Geometry check sheet. Reference: the model listing, model coordinates, mm. A direction names the side the tool comes from. Coordinates: 2 decimals unless noted, no trailing zeros. Write each loop counter-clockwise with the first axis right and the second up, starting at its lowest first coordinate (ties: lowest second). Pieces come first, ordered by that corner, then holes. Notation, with made-up numbers: (78, -26.75) -> (124, -26.75) arc R18 ccw to (124, -8.75) -> close; hole circle Ø3 at (26.5, 67.25). An arc over 180 degrees is marked (long way). Answer as CSV lines item,"result".
```python
from build123d import *

# Parameters (mm, degrees)
SKETCH1_W           = 42
SKETCH1_H           = 20
BOSS_EXTRUDE1_DEPTH = 42
SKETCH2_W           = 55
SKETCH2_H           = 3
BOSS_EXTRUDE2_DEPTH = 20
SKETCH3_R           = 1
CUT_EXTRUDE1_DEPTH  = 42
SKETCH4_R           = 3
BOSS_EXTRUDE3_DEPTH = 5


with BuildPart() as part:
    # Sketch1 → Boss-Extrude1 (new body)
    with BuildSketch(Plane(origin=(0, 0, 0), x_dir=(1, 0, 0), z_dir=(0, 1, 0))):
        with Locations((21, 10)):
            Rectangle(SKETCH1_W, SKETCH1_H)
    extrude(amount=BOSS_EXTRUDE1_DEPTH)

    # Sketch2 → Boss-Extrude2 (add)
    with BuildSketch(Plane.XY):
        with Locations((21, 31.5)):
            Rectangle(SKETCH2_W, SKETCH2_H)
    extrude(amount=-BOSS_EXTRUDE2_DEPTH)

    # Sketch3 → Cut-Extrude1 (cut)
    with BuildSketch(Plane(origin=(0, 33, 0), x_dir=(1, 0, 0), z_dir=(0, 1, 0))):
        with Locations(Location((-4, 15, 0), (0, 0, 270))):
            Circle(SKETCH3_R)
        with Locations(Location((-4, 5, 0), (0, 0, 270))):
            Circle(SKETCH3_R)
        with Locations(Location((46, 15, 0), (0, 0, 270))):
            Circle(SKETCH3_R)
        with Locations(Location((46, 5, 0), (0, 0, 270))):
            Circle(SKETCH3_R)
    extrude(amount=-CUT_EXTRUDE1_DEPTH, mode=Mode.SUBTRACT)

    # Sketch4 → Boss-Extrude3 (add)
    with BuildSketch(Plane(origin=(0, 42, 0), x_dir=(1, 0, 0), z_dir=(0, 1, 0))):
        with Locations(Location((32, 10, 0), (0, 0, 90))):
            Circle(SKETCH4_R)
    extrude(amount=BOSS_EXTRUDE3_DEPTH)


solid = part.part
```
Item 1: Thickness scan on probe 1 along X at (y, z) = (31.85, -15); probe 2 along Y at (x, z) = (34, -1.75). Record the ranges inside material, lowest first.
Responses:
probe 1,"x = -6.5 to -5, -3 to 45, 47 to 48.5"
probe 2,"y = 0 to 42"
Item 2: Release check for a two-part mould opening along X. For faces 5 (the cylindrical face through (-4, 32, -14)), 6 (the flat face through (42, 37, -10)), 7 (the flat face through (-3, 33, -10)) record: +X half, -X half, draft (parallel to the pull), parting line (faces both ways), or undercut.
Responses:
face 5,"undercut"
face 6,"+X half"
face 7,"draft"
Item 3: Cross-section at C-C, the plane z = -10. Record the cut outline in (x, y), plus the area to 3 significant figures.
Responses:
outline,"(-6.5, 30) -> (0, 30) -> (0, 0) -> (42, 0) -> (42, 30) -> (48.5, 30) -> (48.5, 33) -> (42, 33) -> (42, 42) -> (35, 42) -> (35, 47) -> (29, 47) -> (29, 42) -> (0, 42) -> (0, 33) -> (-6.5, 33) -> close"
area,"1,830 mm2"
Item 4: Cross-section at B-B, the plane x = 46. Record the cut outline in (y, z), plus the area to 3 significant figures.
Responses:
outline,"(30, -20) -> (33, -20) -> (33, -16) -> (30, -16) -> close; (30, -14) -> (33, -14) -> (33, -6) -> (30, -6) -> close; (30, -4) -> (33, -4) -> (33, 0) -> (30, 0) -> close"
area,"48.0 mm2"
Item 5: Depth check by flat-ended pin: pin 1 Ø1 at (y, z) = (14, -18) entering from +X; pin 2 Ø6 at (y, z) = (14, -5.5) entering from -X; pin 3 Ø7 at (x, z) = (-4, -11) entering from -Y; pin 4 Ø1.8 at (x, z) = (46, -15) entering from +Y. Enter the tip coordinate at first touch or a pass-through.
Responses:
pin 1,"stops at x = 42"
pin 2,"stops at x = 0"
pin 3,"stops at y = 30"
pin 4,"passes through"
Item 6: Cross-section at D-D, the plane y = 37. Record the cut outline in (x, z), plus the area to 3 significant figures.
Responses:
outline,"(0, -20) -> (42, -20) -> (42, 0) -> (0, 0) -> close"
area,"840 mm2"
Item 7: Set-up check for faces 1 (the flat face through (0, 37, -10)), 2 (the flat face through (-3, 30, -10)), 3 (the flat face through (42, 15, -10)), 4 (the flat face through (45, 33, -10)): record each of +Z, -Z, +X, -X, +Y, -Y from which the full face is reachable in a straight line by a thin tool's end or side.
Responses:
face 1,"+Z, -Z, -X, +Y"
face 2,"+Z, -Z, -X, -Y"
face 3,"+Z, -Z, +X, -Y"
face 4,"+Z, -Z, +X, +Y"
Item 8: Cross-section at A-A, the plane z = -15. Record the cut outline in (x, y), plus the area to 3 significant figures.
Responses:
outline,"(-6.5, 30) -> (-5, 30) -> (-5, 33) -> (-6.5, 33) -> close; (-3, 30) -> (0, 30) -> (0, 0) -> (42, 0) -> (42, 30) -> (45, 30) -> (45, 33) -> (42, 33) -> (42, 42) -> (0, 42) -> (0, 33) -> (-3, 33) -> close; (47, 30) -> (48.5, 30) -> (48.5, 33) -> (47, 33) -> close"
area,"1,790 mm2"
